```python
from build123d import *

# Parameters (mm, degrees)
SKETCH_1_W                    = 67
SKETCH_1_H                    = 19
EXTRUDE_1_DEPTH               = 89
CUT_EXTRUDE_1_DEPTH           = 96.56934655
CUT_EXTRUDE_2_REACH           = 98.976
SKETCH_3_W                    = 57
SKETCH_3_H                    = 7
SKETCH_3_H_2                  = 40
SKETCH_4_W                    = 8.5
SKETCH_4_H                    = 23
CUT_EXTRUDE_3_DEPTH           = 12
HOLE_WIZARD_1_4_201_D         = 5.1054
HOLE_WIZARD_3_8_161_D         = 7.9375
HOLE_WIZARD_3_8_161_DEPTH     = 26.99
HOLE_WIZARD_3_8_161_TIP       = 2.384665582
FILLET_1_R                    = 1
HOLE_START                    = -41.5
HOLE_WIZARD_3_8_162_OUTLINE_R = 3.96875
HOLE_WIZARD_3_8_162_DEPTH     = 13
HOLE_WIZARD_1_4_202_REACH     = 118.774
HOLE_WIZARD_1_4_202_BORE_R    = 2.5527
SKETCH_17_R                   = 3.5
EXTRUDE_2_DEPTH               = 7
FILLET_2_R                    = 1
CHAMFER_1_SIZE                = 0.5
CUT_EXTRUDE_4_DEPTH           = 33
SKETCH_19_R                   = 5.5
EXTRUDE_3_DEPTH               = 1


with BuildPart() as part:
    # Эскиз1 → Бобышка-Вытянуть1 (new body)
    with BuildSketch(Plane.XY):
        Rectangle(SKETCH_1_W, SKETCH_1_H)
    extrude(amount=EXTRUDE_1_DEPTH)

    # Эскиз2 → Вырез-Вытянуть1 (cut, through all)
    with BuildSketch(Plane.XY.offset(89)):
        Polygon((-28.5, 2.5), (28.5, 2.5), (28.5, 3.5), (25.75, 8.263139721), (25.75, 9.5), (-25.75, 9.5), (-25.75, 8.263139721), (-28.5, 3.5), align=None)
    extrude(amount=-CUT_EXTRUDE_1_DEPTH, mode=Mode.SUBTRACT)

    # Вырез-Вытянуть2: up to this face of the body (flat: up to its plane)
    cut_extrude_2_end = Plane(part.part.faces().sort_by_distance((0, 2.5, 44.5))[0])
    # Эскиз3 → Вырез-Вытянуть2 (cut, up to the picked face)
    with BuildSketch(Plane(origin=(0, 9.5, 0), x_dir=(1, 0, 0), z_dir=(0, 1, 0)), mode=Mode.PRIVATE) as cut_extrude_2_sk1:
        with Locations((0, -85.5)):
            Rectangle(SKETCH_3_W, SKETCH_3_H)
    cut_extrude_2_tool1 = split(extrude(cut_extrude_2_sk1.sketch, amount=-CUT_EXTRUDE_2_REACH, mode=Mode.PRIVATE), bisect_by=cut_extrude_2_end, keep=Keep.BOTH, mode=Mode.PRIVATE)
    # Эскиз3 → Вырез-Вытянуть2 (cut, up to the picked face)
    with BuildSketch(Plane(origin=(0, 9.5, 0), x_dir=(1, 0, 0), z_dir=(0, 1, 0)), mode=Mode.PRIVATE) as cut_extrude_2_sk2:
        with Locations((0, -44.5)):
            Rectangle(SKETCH_3_W, SKETCH_3_H_2)
    cut_extrude_2_tool2 = split(extrude(cut_extrude_2_sk2.sketch, amount=-CUT_EXTRUDE_2_REACH, mode=Mode.PRIVATE), bisect_by=cut_extrude_2_end, keep=Keep.BOTH, mode=Mode.PRIVATE)
    # Эскиз3 → Вырез-Вытянуть2 (cut, up to the picked face)
    with BuildSketch(Plane(origin=(0, 9.5, 0), x_dir=(1, 0, 0), z_dir=(0, 1, 0)), mode=Mode.PRIVATE) as cut_extrude_2_sk3:
        with Locations((0, -3.5)):
            Rectangle(SKETCH_3_W, SKETCH_3_H)
    cut_extrude_2_tool3 = split(extrude(cut_extrude_2_sk3.sketch, amount=-CUT_EXTRUDE_2_REACH, mode=Mode.PRIVATE), bisect_by=cut_extrude_2_end, keep=Keep.BOTH, mode=Mode.PRIVATE)
    add(cut_extrude_2_tool1.solids().sort_by(Axis((0, 9.5, 85.5), (0, -1, 0)))[0], mode=Mode.SUBTRACT)
    add(cut_extrude_2_tool2.solids().sort_by(Axis((0, 9.5, 44.5), (0, -1, 0)))[0], mode=Mode.SUBTRACT)
    add(cut_extrude_2_tool3.solids().sort_by(Axis((0, 9.5, 3.5), (0, -1, 0)))[0], mode=Mode.SUBTRACT)

    # Эскиз4 → Вырез-Вытянуть3 (cut)
    with BuildSketch(Plane.XZ.offset(9.5)):
        with Locations((-24.25, 72.5)):
            Rectangle(SKETCH_4_W, SKETCH_4_H)
        with Locations((24.25, 72.5)):
            Rectangle(SKETCH_4_W, SKETCH_4_H)
        with Locations((-24.25, 16.5)):
            Rectangle(SKETCH_4_W, SKETCH_4_H)
        with Locations((24.25, 16.5)):
            Rectangle(SKETCH_4_W, SKETCH_4_H)
    extrude(amount=-CUT_EXTRUDE_3_DEPTH, mode=Mode.SUBTRACT)

    # Отверстие обработанное метчиком 1/4-201 (through all)
    with Locations(Plane(origin=(0, -9.5, 0), x_dir=(-1, 0, 0), z_dir=(0, -1, 0))):
        with Locations((0, -36)):
            Hole(HOLE_WIZARD_1_4_201_D / 2)

    # Отверстие обработанное метчиком 3/8-161
    with Locations(Plane(origin=(0, -9.5, 0), x_dir=(-1, 0, 0), z_dir=(0, -1, 0))):
        with Locations((0, -53)):
            Hole(HOLE_WIZARD_3_8_161_D / 2, depth=HOLE_WIZARD_3_8_161_DEPTH)
            with Locations((0, 0, -(HOLE_WIZARD_3_8_161_DEPTH + HOLE_WIZARD_3_8_161_TIP / 2))):  # 118° drill point
                Cone(0, HOLE_WIZARD_3_8_161_D / 2, HOLE_WIZARD_3_8_161_TIP, mode=Mode.SUBTRACT)

    # Скругление1
    fillet_1_edges = [part.edges().sort_by_distance(p)[0] for p in [
        (-20, -3.5, 84),
        (-20, -3.5, 61),
        (-28.5, -3.5, 61),
        (-28.5, -3.5, 84),
        (20, -3.5, 84),
        (28.5, -3.5, 84),
        (28.5, -3.5, 61),
        (20, -3.5, 61),
        (-28.5, -3.5, 5),
        (-28.5, -3.5, 28),
        (-20, -3.5, 28),
        (-20, -3.5, 5),
        (28.5, -3.5, 28),
        (28.5, -3.5, 5),
        (20, -3.5, 5),
        (20, -3.5, 28),
    ]]
    fillet(fillet_1_edges, radius=FILLET_1_R)

    # По сечениям1: read off the stored shape, not the designer's step
    # По сечениям1: loft between two sections, ruled curve by curve
    loft_1_from = [
        Edge.make_bspline([(-33.5, 5.960828972, 20.335589749), (-33.5, 16.63200847, 8.413931805), (-33.5, 4.710350526, -2.257247693), (-33.5, -5.960828972, 9.664410251), (-33.5, -16.63200847, 21.586068195), (-33.5, -4.710350526, 32.257247693), (-33.5, 5.960828972, 20.335589749)], [0, 0, 0, 0, 0.5, 0.5, 0.5, 1, 1, 1, 1], 3, [1, 0.333333333, 0.333333333, 1, 0.333333333, 0.333333333, 1]),
    ]
    loft_1_to = [
        Edge.make_bspline([(-41.5, 5.342611917, 17.730658877), (-41.5, 10.803929671, 7.045435042), (-41.5, 0.118705836, 1.584117289), (-41.5, -5.342611917, 12.269341123), (-41.5, -10.803929671, 22.954564958), (-41.5, -0.118705836, 28.415882711), (-41.5, 5.342611917, 17.730658877)], [0, 0, 0, 0, 0.5, 0.5, 0.5, 1, 1, 1, 1], 3, [1, 0.333333333, 0.333333333, 1, 0.333333333, 0.333333333, 1]),
    ]
    loft_1 = Solid(Shell([*[Face.make_surface_from_curves(loft_1_from[k], loft_1_to[k]) for k in range(1)], Face(Wire(loft_1_from)), Face(Wire(loft_1_to))]))
    add(loft_1)

    # Зеркальное отражение1: По сечениям1 across plane
    add(loft_1.mirror(Plane.XY.offset(44.5)))

    # Отверстие обработанное метчиком 3/8-162: read off the stored shape, not the designer's step
    # Отверстие обработанное метчиком 3/8-162 outline → Отверстие обработанное метчиком 3/8-162 (cut)
    with BuildSketch(Plane.YZ.offset(HOLE_START)):
        with Locations((0, 74)):
            Circle(HOLE_WIZARD_3_8_162_OUTLINE_R)
    extrude(amount=HOLE_WIZARD_3_8_162_DEPTH, mode=Mode.SUBTRACT)

    # Отверстие обработанное метчиком 1/4-202 bore → Отверстие обработанное метчиком 1/4-202 (cut, up to next)
    with BuildSketch(Plane.ZY.offset(41.5), mode=Mode.PRIVATE) as hole_wizard_1_4_202_sk1:
        with Locations((15, 0)):
            Circle(HOLE_WIZARD_1_4_202_BORE_R)
    hole_wizard_1_4_202_tool1 = extrude(hole_wizard_1_4_202_sk1.sketch, amount=-HOLE_WIZARD_1_4_202_REACH, mode=Mode.PRIVATE) & part.part
    add(hole_wizard_1_4_202_tool1.solids().sort_by_distance((-41.5, 0, 15))[0], mode=Mode.SUBTRACT)

    # Эскиз17 → Бобышка-Вытянуть2 (add)
    with BuildSketch(Plane.ZY.offset(33.5)):
        with Locations(Location((44.5, -2.5, 0), (0, 0, 180))):
            Circle(SKETCH_17_R)
    extrude(amount=EXTRUDE_2_DEPTH)

    # Скругление2
    fillet_2_edges = [part.edges().sort_by_distance(p)[0] for p in [
        (-41.5, -5.342611917, 12.269341123),
        (-33.5, -5.960828972, 9.664410251),
        (-33.5, -5.960828972, 79.335589749),
        (-41.5, -5.342611917, 76.730658877),
    ]]
    fillet(fillet_2_edges, radius=FILLET_2_R)

    # Фаска1
    chamfer_1_edges = [part.edges().sort_by_distance(p)[0] for p in [
        (-40.5, -2.5, 48),
    ]]
    chamfer(chamfer_1_edges, length=CHAMFER_1_SIZE)

    # Эскиз18 → Вырез-Вытянуть4 (cut)
    with BuildSketch(Plane(origin=(16.5, 0, 0), x_dir=(0, 0, -1), z_dir=(1, 0, 0))):
        Polygon((-89, -1.5), (-89, 2.5), (-74, 2.5), align=None)
    cut_extrude_4 = extrude(amount=-CUT_EXTRUDE_4_DEPTH, mode=Mode.SUBTRACT)

    # Зеркальное отражение2: Вырез-Вытянуть4 across plane
    add(cut_extrude_4.mirror(Plane.XY.offset(44.5)), mode=Mode.SUBTRACT)

    # Эскиз19 → Бобышка-Вытянуть3 (add)
    with BuildSketch(Plane(origin=(33.5, 0, 0), x_dir=(0, 0, -1), z_dir=(1, 0, 0))):
        with Locations(Location((-44.5, -2.5, 0), (0, 0, 180))):
            Circle(SKETCH_19_R)
    extrude(amount=EXTRUDE_3_DEPTH)


solid = part.part
```
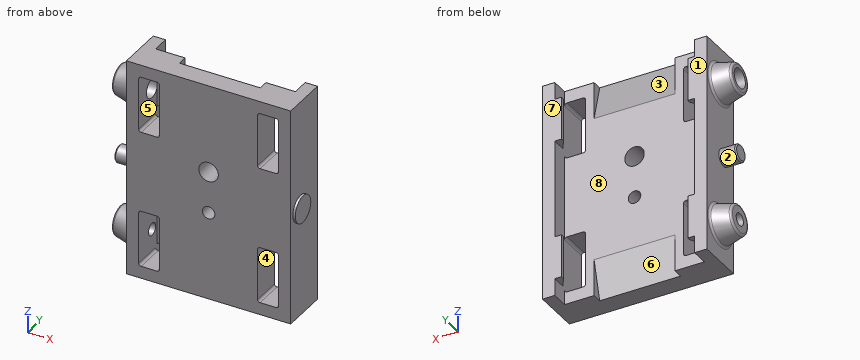
CAD build for the part. Positions are in the model's coordinates, mm. Face numbers are marked on the shaded views. A direction names the side the tool comes from. Round coordinates to 2 decimals unless told otherwise and drop trailing zeros. Write each loop counter-clockwise with the first axis right and the second up, starting at its lowest first coordinate (ties: lowest second). Pieces come first, ordered by that corner, then holes. Notation, with made-up numbers: (-37.5, 71.25) - (13.5, 71.25) arc R19 cw to (13.5, 76.25) - close; hole circle Ø11 at (9, 65). An arc over 180 degrees is marked (long way). Return JSON: item names as keys, results as strings. Group by question number.
Item 1: Mould opens along Z. For the marked faces 1, 2 and 3 say: +Z half, -Z half, draft (parallel to the pull), parting line (faces both ways), or undercut.
Item 2: Probe probe 1 along Z at (x, y) = (-24, -3.5); probe 2 along X at (y, z) = (-2, 18); probe 3 along X at (y, z) = (5.75, 52.5). List the from-to ranges inside material, lowest first.
Item 3: Band-saw the part on B-B on z = 36. List the corners of the cut face in (x, y), plus the area to 3 significant figures.
Item 4: Band-saw the part on C-C on x = 11.5. List the corners of the cut face in (y, z).
Item 5: Flat gauge pins, fed straight in: pin 1 Ø10 at (y, z) = (-4.5, 52) entering from -X; pin 2 Ø6 at (y, z) = (3, 60) entering from +X; pin 3 Ø0.8 at (x, y) = (-27, 7.5) entering from -Z. Where does each tip first touch, or does it go through?
Item 6: 3-axis set-ups, long thin cutter, end or side, ignore diameter. For the marked faces 4, 5, 6, 7 and 8: which of +Z, -Z, +X, -X, +Y, -Y reach the whole face in a straight line?
Item 7: Band-saw the part on A-A on x = 0. List the corners of the cut face in (y, z).
Resolved:
{
 "1": {"face 1": "draft", "face 2": "undercut", "face 3": "+Z half"},
 "2": {"probe 1": "z = 0 to 5, 28 to 61, 84 to 89", "probe 2": "x = -41.5 to -28.5, -20 to 20, 28.5 to 33.5", "probe 3": "x = -33.5 to -28.5, 28.5 to 33.5"},
 "3": {"outline": "(-33.5, -9.5) - (-2.55, -9.5) - (-2.55, 2.5) - (-28.5, 2.5) - (-28.5, 9.5) - (-33.5, 9.5) - close; (2.55, -9.5) - (33.5, -9.5) - (33.5, 9.5) - (28.5, 9.5) - (28.5, 2.5) - (2.55, 2.5) - close", "area": "813 mm²"},
 "4": {"outline": "(-9.5, 0) - (-1.5, 0) - (2.5, 15) - (2.5, 74) - (-1.5, 89) - (-9.5, 89) - close"},
 "5": {"pin 1": "stops at x = -40.5", "pin 2": "stops at x = 33.5", "pin 3": "stops at z = 7"},
 "6": {"face 4": "+Y, -Y", "face 5": "none", "face 6": "-Z, +Y", "face 7": "+Z, -Z, +X, -X, +Y", "face 8": "+Z, -Z, +Y"},
 "7": {"outline": "(-9.5, 0) - (-1.5, 0) - (2.5, 15) - (2.5, 33.45) - (-9.5, 33.45) - close; (-9.5, 38.55) - (2.5, 38.55) - (2.5, 49.03) - (-9.5, 49.03) - close; (-9.5, 56.97) - (2.5, 56.97) - (2.5, 74) - (-1.5, 89) - (-9.5, 89) - close"}
}
